Model file for the job. Use its own axes, mm. A direction names the side the tool comes from. Round coordinates to 2 decimals unless told otherwise and drop trailing zeros. Loops run counter-clockwise (first coordinate to the right, second up) from the corner with the lowest first, then second, coordinate; pieces in that order, holes last. Notation, with made-up numbers: (-22.75, 31.25) -> (-10.75, 31.25) arc R21 cw to (-10.75, 63.25) -> close; hole circle Ø10 at (82.25, 61.25). An arc over 180 degrees is marked (long way). Use a Markdown table: item, result.
from build123d import *

# Parameters (mm, degrees)
SKETCH1_W           = 50.8
SKETCH1_H           = 50.8
SKETCH1_R           = 2
SKETCH1_W_2         = 5
SKETCH1_H_2         = 5
BOSS_EXTRUDE1_DEPTH = 5
FILLET1_R           = 2
FILLET2_R           = 4.54
SKETCH1_6_W         = 5
SKETCH1_6_H         = 5
BOSS_EXTRUDE2_DEPTH = 12


with BuildPart() as part:
    # Sketch1 → Boss-Extrude1 (new body)
    with BuildSketch(Plane(origin=(0, 0, 0), x_dir=(1, 0, 0), z_dir=(0, 1, 0))):
        Rectangle(SKETCH1_W, SKETCH1_H)
        with Locations(Location((0, 0, 0), (0, 0, 270))):
            Circle(SKETCH1_R, mode=Mode.SUBTRACT)
        with Locations((-19.4, 19.4)):
            Rectangle(SKETCH1_W_2, SKETCH1_H_2, mode=Mode.SUBTRACT)
        with Locations((19.4, 19.4)):
            Rectangle(SKETCH1_W_2, SKETCH1_H_2, mode=Mode.SUBTRACT)
        with Locations((-19.4, -19.4)):
            Rectangle(SKETCH1_W_2, SKETCH1_H_2, mode=Mode.SUBTRACT)
        with Locations((19.4, -19.4)):
            Rectangle(SKETCH1_W_2, SKETCH1_H_2, mode=Mode.SUBTRACT)
    extrude(amount=BOSS_EXTRUDE1_DEPTH)

    # Fillet1
    fillet1_edges = [part.edges().sort_by_distance(p)[0] for p in [
        (0, 0, 25.4),
        (-25.4, 0, 0),
        (0, 0, -25.4),
        (25.4, 0, 0),
    ]]
    fillet(fillet1_edges, radius=FILLET1_R)

    # Fillet2
    # the kernel refuses this fillet: 4.54 mm, written as the material it takes off along each edge
    with BuildSketch(Plane(origin=(20.86, 0, -20.86), x_dir=(0, 0, -1), z_dir=(-1, 0, 0))) as fillet2_piece_1:
        with BuildLine():
            CenterArc((2.54, -2), 2, 0, 90)
            Line((4.54, -2), (4.54, 0))
            Line((4.54, 0), (2.54, 0))
        make_face()
    revolve(axis=Axis((20.86, 0, -20.86), (0, -1, 0)), revolution_arc=90, mode=Mode.SUBTRACT)
    with BuildSketch(Plane(origin=(20.86, 0, 20.86), x_dir=(1, 0, 0), z_dir=(0, 0, -1))) as fillet2_piece_2:
        with BuildLine():
            CenterArc((2.54, -2), 2, 0, 90)
            Line((4.54, -2), (4.54, 0))
            Line((4.54, 0), (2.54, 0))
        make_face()
    revolve(axis=Axis((20.86, 0, 20.86), (0, -1, 0)), revolution_arc=90, mode=Mode.SUBTRACT)
    with BuildSketch(Plane(origin=(-20.86, 0, -20.86), x_dir=(-1, 0, 0), z_dir=(0, 0, 1))) as fillet2_piece_3:
        with BuildLine():
            CenterArc((2.54, -2), 2, 0, 90)
            Line((4.54, -2), (4.54, 0))
            Line((4.54, 0), (2.54, 0))
        make_face()
    revolve(axis=Axis((-20.86, 0, -20.86), (0, -1, 0)), revolution_arc=90, mode=Mode.SUBTRACT)
    with BuildSketch(Plane(origin=(-20.86, 0, 20.86), x_dir=(0, 0, 1), z_dir=(1, 0, 0))) as fillet2_piece_4:
        with BuildLine():
            CenterArc((2.54, -2), 2, 0, 90)
            Line((4.54, -2), (4.54, 0))
            Line((4.54, 0), (2.54, 0))
        make_face()
    revolve(axis=Axis((-20.86, 0, 20.86), (0, -1, 0)), revolution_arc=90, mode=Mode.SUBTRACT)
    with BuildSketch(Plane(origin=(25.4, 0, 25.4), x_dir=(0, 0, -1), z_dir=(0, 1, 0)), Plane(origin=(25.4, 0, -25.4), x_dir=(-1, 0, 0), z_dir=(0, 1, 0))) as fillet2_piece_5:
        with BuildLine():
            CenterArc((FILLET2_R, FILLET2_R), FILLET2_R, 180, 90)
            Line((0, FILLET2_R), (0, 0))
            Line((0, 0), (FILLET2_R, 0))
        make_face()
    extrude(amount=16.35, mode=Mode.SUBTRACT)
    with BuildSketch(Plane(origin=(-25.4, 0, 25.4), x_dir=(0, 0, -1), z_dir=(0, 1, 0)), Plane(origin=(-25.4, 0, -25.4), x_dir=(1, 0, 0), z_dir=(0, 1, 0))) as fillet2_piece_6:
        with BuildLine():
            CenterArc((FILLET2_R, -FILLET2_R), FILLET2_R, 90, 90)
            Line((0, -FILLET2_R), (0, 0))
            Line((0, 0), (FILLET2_R, 0))
        make_face()
    extrude(amount=16.35, mode=Mode.SUBTRACT)

    # Sketch1<6> → Boss-Extrude2 (add)
    with BuildSketch(Plane(origin=(0, 0, 0), x_dir=(1, 0, 0), z_dir=(0, 1, 0))):
        with Locations((-19.4, -19.4)):
            Rectangle(SKETCH1_6_W, SKETCH1_6_H)
        with Locations((19.4, -19.4)):
            Rectangle(SKETCH1_6_W, SKETCH1_6_H)
        with Locations((19.4, 19.4)):
            Rectangle(SKETCH1_6_W, SKETCH1_6_H)
        with Locations((-19.4, 19.4)):
            Rectangle(SKETCH1_6_W, SKETCH1_6_H)
    extrude(amount=BOSS_EXTRUDE2_DEPTH)


solid = part.part
Q1. Band-saw the part on B-B, the plane y = 7. Give the cut face in (x, z).
Results list:
| item | result |
|---|---|
| outline | (-21.9, -21.9) -> (-16.9, -21.9) -> (-16.9, -16.9) -> (-21.9, -16.9) -> close; (-21.9, 16.9) -> (-16.9, 16.9) -> (-16.9, 21.9) -> (-21.9, 21.9) -> close; (16.9, -21.9) -> (21.9, -21.9) -> (21.9, -16.9) -> (16.9, -16.9) -> close; (16.9, 16.9) -> (21.9, 16.9) -> (21.9, 21.9) -> (16.9, 21.9) -> close |
Q2. Band-saw the part on A-A, the plane x = 0. Give the cut face in (y, z).
Results list:
| item | result |
|---|---|
| outline | (0, -23.4) arc R2 ccw to (2, -25.4) -> (5, -25.4) -> (5, -2) -> (0, -2) -> close; (0, 2) -> (5, 2) -> (5, 25.4) -> (2, 25.4) arc R2 ccw to (0, 23.4) -> close |
Q3. Drill centre lines: L1, parallel to X at y = 3.1, z = 0; L2, parallel to X at y = 7.25, z = -20.5; L3, parallel to Y at x = -19, z = -12.5. Where is each one in solid material? Low to high. Write a range as from..to.
Results list:
| item | result |
|---|---|
| L1 | x = -25.4..-2, 2..25.4 |
| L2 | x = -21.9..-16.9, 16.9..21.9 |
| L3 | y = 0..5 |
Q4. Pull direction Z, two halves, no side cores. Call faces 1 (the face through (19, 8, 21.9)), 2 (the face through (0, 0, -6)), 3 (the face through (19, 8, -16.9)): released by +Z, released by -Z, zero draft, split by the parting line, or undercut.
Results list:
| item | result |
|---|---|
| face 1 | released by +Z |
| face 2 | zero draft |
| face 3 | undercut |
Q5. Band-saw the part on C-C, the plane z = 0. Give the cut face in (x, y), plus the area to 3 significant figures.
Results list:
| item | result |
|---|---|
| outline | (-25.4, 2) arc R2 ccw to (-23.4, 0) -> (-2, 0) -> (-2, 5) -> (-25.4, 5) -> close; (2, 0) -> (23.4, 0) arc R2 ccw to (25.4, 2) -> (25.4, 5) -> (2, 5) -> close |
| area | 232 mm² |
Q6. Flat gauge pins, fed straight in: pin 1 (2.5 mm diameter, centred on y = 8.5, z = -18.5, fed in from +X); pin 2 (5.5 mm diameter, centred on y = 9, z = 20.5, fed in from -X); pin 3 (4 mm diameter, centred on x = 3.5, z = 19, fed in from +Y); pin 4 (3.5 mm diameter, centred on x = 0, z = 0, fed in from +Y). Where does each tip first touch, or does it go through?
Results list:
| item | result |
|---|---|
| pin 1 | stops at x = 21.9 |
| pin 2 | stops at x = -21.9 |
| pin 3 | stops at y = 5 |
| pin 4 | passes through |
Q7. Band-saw the part on D-D, the plane y = 1.25. Give the cut face in (x, z), plus the area to 3 significant figures.
Results list:
| item | result |
|---|---|
| outline | (-25.25, -20.86) arc R4.39 ccw to (-20.86, -25.25) -> (20.86, -25.25) arc R4.39 ccw to (25.25, -20.86) -> (25.25, 20.86) arc R4.39 ccw to (20.86, 25.25) -> (-20.86, 25.25) arc R4.39 ccw to (-25.25, 20.86) -> close; hole circle Ø4 at (0, 0) |
| area | 2,520 mm² |
Q8. Tool access for faces 4 (the face through (-19, 8, 16.9)), 5 (the face through (-16.9, 8, -19)), 6 (the face through (-19, 8, 21.9)), 7 (the face through (21.9, 8, 19)): list every direction of +Z, -Z, +X, -X, +Y, -Y with a clear straight run to the whole face (end or side of a thin tool).
Results list:
| item | result |
|---|---|
| face 4 | +X, -X, +Y |
| face 5 | +Z, -Z, +Y |
| face 6 | +Z, +X, -X, +Y |
| face 7 | +Z, -Z, +X, +Y |
